Solid Edge part; units mm, degrees
sketch "Sketch1" plane through (0, 0, 0) normal (0, 0, 1) x (1, 0, 0)
  line L0 (-7.25, -45) -> (7.25, -45)
  line L1 (7.25, -45) -> (7.25, 45)
  line L2 (7.25, 45) -> (-7.25, 45)
  line L3 (-7.25, 45) -> (-7.25, -45)
  dimension "D1" = 7.25
  dimension "D2" = 7.25
extrude "Protrusion1" add sketch "Sketch1" along normal blind 12
sketch "Sketch2" plane through (0, 0, 0) normal (0, 0, -1) x (0, -1, 0)
  circle A0 centre (-26.5, 0) radius 2.1
  circle A1 centre (-37.5, 0) radius 3.1
  circle A2 centre (-15, 0) radius 3.1
extrude "Cutout1" cut sketch "Sketch2" against normal up to next
sketch "Sketch3" plane through (0, 0, 0) normal (0, 0, -1) x (0, -1, 0)
  circle A0 centre (-15, 0) radius 5.1
  circle A1 centre (-26.5, 0) radius 3.6
extrude "ExtrudedCutout_2" cut sketch "Sketch3" against normal blind 8
sketch "Sketch4" plane through (0, 0, 12) normal (0, 0, 1) x (0, -1, 0)
  circle A0 centre (-37.5, 0) radius 5.1
extrude "ExtrudedCutout_3" cut sketch "Sketch4" against normal blind 8
mirror "Mirror1" about plane through (0, 0, 0) normal (0, 1, 0) of "Cutout1", "ExtrudedCutout_2", "ExtrudedCutout_3"
Could you check a few things on this model? Use its own coordinates, in mm. A direction names the side the tool comes from. Round coordinates to 2 decimals unless told otherwise and drop trailing zeros. Write each loop counter-clockwise with the first axis right and the second up, starting at its lowest first coordinate (ties: lowest second). Pieces come first, ordered by that corner, then holes. Notation, with made-up numbers: M 50,23 L 62,23 A36 ccw 62,62 Z; hole C 37.5,49.25 d2. An arc over 180 degrees is marked long. Write each question's results on one line, items separated by ' | '. Start each with the question number.
1. I need wall thicknesses on L1, parallel to Y at x = 4.5, z = 2.5; L2, parallel to X at y = 15, z = 2.75; L3, parallel to Y at x = -3.25, z = 2.5. Which ranges of each line are inside material? Lowest first, please. Write a range as from..to.
2. Imagine slicing it at C-C on y = 15. List the corners of the cut face in (x, z) for me, and give its area (3 significant figures).
3. Imagine slicing it at A-A on y = 26.5. List the corners of the cut face in (x, z) for me.
4. Imagine slicing it at B-B on z = 11.25. List the corners of the cut face in (x, y) for me.
5. Thinking about a two-plate mould opening in X: for faces 4 (the face through (0, -45, 6)), 5 (the face through (-0.224, -42.595, 8.056)), 6 (the face through (7.25, -1, 6)), which applies, +X half, -X half, draft (parallel to the pull), parting line (faces both ways), or undercut?
6. I'm going to push flat-ended pins straight in: pin 1 Ø5 at (x, y) = (-1.5, -35.5) entering from +Z; pin 2 Ø5.5 at (x, y) = (0, -15) entering from +Z; pin 3 Ø3.5 at (x, y) = (0.5, 27) entering from -Z. Where does each tip first touch, or does it pass through?
7. On a 3-axis mill with a long thin cutter (end or side, diameter ignored), from which of +Z, -Z, +X, -X, +Y, -Y can I reach the whole of each face in a straight line? I mean faces 1 (the face through (-7.25, 1, 6)), 2 (the face through (0.224, 42.595, 8.056)), 3 (the face through (2, -25, 8)). Say none if no direction works.
Result sheet:
1) L1: y = -45..-17.4, -12.6..12.6, 17.4..45 | L2: x = -7.25..-5.1, 5.1..7.25 | L3: y = -45..-28.05, -24.95..-18.93, -11.07..11.07, 18.93..24.95, 28.05..45
2) outline: M -7.25,0 L -5.1,0 L -5.1,8 L -3.1,8 L -3.1,12 L -7.25,12 Z; M 3.1,8 L 5.1,8 L 5.1,0 L 7.25,0 L 7.25,12 L 3.1,12 Z | area: 67.6 mm^2
3) outline: M -7.25,0 L -3.6,0 L -3.6,8 L -2.1,8 L -2.1,12 L -7.25,12 Z; M 2.1,8 L 3.6,8 L 3.6,0 L 7.25,0 L 7.25,12 L 2.1,12 Z
4) outline: M -7.25,-45 L 7.25,-45 L 7.25,45 L -7.25,45 Z; hole C 0,-37.5 d10.2; hole C 0,37.5 d10.2; hole C 0,-15 d6.2; hole C 0,15 d6.2; hole C 0,-26.5 d4.2; hole C 0,26.5 d4.2
5) face 4: draft | face 5: undercut | face 6: +X half
6) pin 1: stops at z = 4 | pin 2: passes through | pin 3: stops at z = 8
7) face 1: +Z, -Z, -X, +Y, -Y | face 2: +Z | face 3: -Z
